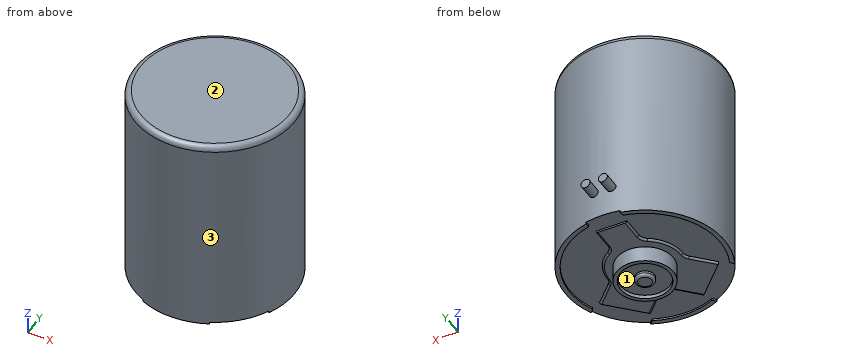
from build123d import *

# Parameters (mm, degrees)
SKETCH_1_R          = 21.05
EXTRUDE_1_DEPTH     = 53.3
FILLET_1_R          = 1.5
CUT_EXTRUDE_1_DEPTH = 0.5
SKETCH_3_R          = 7.5
EXTRUDE_2_DEPTH     = 4.2
SKETCH_4_R          = 6.5
CUT_EXTRUDE_2_DEPTH = 1
SKETCH_5_R          = 2.5
EXTRUDE_3_DEPTH     = 1.3
FILLET_2_R          = 0.75
FILLET_3_R          = 2.5
FILLET_4_R          = 0.5
SKETCH_7_W          = 9
SKETCH_7_H          = 4.55
CUT_EXTRUDE_3_DEPTH = 0.5
SKETCH_9_R          = 21
EXTRUDE_4_DEPTH     = 39.2
EXTRUDE_5_DEPTH     = 2
SKETCH_11_R         = 8
EXTRUDE_6_DEPTH     = 0.5
SKETCH_12_R         = 7.1
EXTRUDE_7_DEPTH     = 1
SKETCH_13_R         = 4
EXTRUDE_8_DEPTH     = 20
SKETCH_14_W         = 8
SKETCH_14_H         = 12
CUT_EXTRUDE_4_DEPTH = 1
SKETCH_15_R         = 2
CUT_EXTRUDE_5_DEPTH = 6
CHAMFER_1_SIZE      = 0.5
EXTRUDE_9_DEPTH     = 25
CHAMFER_2_SIZE      = 0.2
OTHER_START         = 53.3
OTHER_1_OUTLINE_R   = 21
OTHER_1_DEPTH       = 61.2


# Read off the part's stored shape, not the designer's step: 交差1
with BuildPart() as part:
    # ｽｹｯﾁ1 → ﾎﾞｽ - 押し出し1 (new body)
    with BuildSketch(Plane.XY):
        Circle(SKETCH_1_R)
    extrude(amount=EXTRUDE_1_DEPTH)

    # ﾌｨﾚｯﾄ1
    fillet_1_edges = [part.edges().sort_by_distance(p)[0] for p in [
        (-21.05, 0, 53.3),
    ]]
    fillet(fillet_1_edges, radius=FILLET_1_R)

    # ｽｹｯﾁ2 → ｶｯﾄ - 押し出し1 (cut)
    with BuildSketch(Plane(origin=(0, 0, 0), x_dir=(-1, 0, 0), z_dir=(0, 0, -1))):
        with BuildLine():
            Line((-1.767766953, -10.606601718), (-8.902744604, -17.741579369))
            ThreePointArc((-8.902744604, -17.741579369), (0, -19.85), (8.902744604, -17.741579369))
            Line((8.902744604, -17.741579369), (1.767766953, -10.606601718))
            ThreePointArc((1.767766953, -10.606601718), (0, -9.874368671), (-1.767766953, -10.606601718))
        make_face()
        with BuildLine():
            Line((-17.741579369, -8.902744604), (-9.939267924, -1.100433159))
            ThreePointArc((-9.939267924, -1.100433159), (-8.682968675, 4.960449072), (-4.1, 9.120855223))
            Line((-4.1, 9.120855223), (-4.1, 19.421959221))
            ThreePointArc((-4.1, 19.421959221), (-17.883955352, 8.613166721), (-17.741579369, -8.902744604))
        make_face()
        with BuildLine():
            Line((4.1, 19.421959221), (4.1, 9.120855223))
            ThreePointArc((4.1, 9.120855223), (8.682968675, 4.960449072), (9.939267924, -1.100433159))
            Line((9.939267924, -1.100433159), (17.741579369, -8.902744604))
            ThreePointArc((17.741579369, -8.902744604), (17.883955352, 8.613166721), (4.1, 19.421959221))
        make_face()
    extrude(amount=-CUT_EXTRUDE_1_DEPTH, mode=Mode.SUBTRACT)

    # ｽｹｯﾁ3 → ﾎﾞｽ - 押し出し2 (add)
    with BuildSketch(Plane(origin=(0, 0, 0), x_dir=(-1, 0, 0), z_dir=(0, 0, -1))):
        with Locations(Location((0, 0, 0), (0, 0, 180))):
            Circle(SKETCH_3_R)
    extrude(amount=EXTRUDE_2_DEPTH)

    # ｽｹｯﾁ4 → ｶｯﾄ - 押し出し2 (cut)
    with BuildSketch(Plane(origin=(0, 0, -4.2), x_dir=(-1, 0, 0), z_dir=(0, 0, -1))):
        Circle(SKETCH_4_R)
    extrude(amount=-CUT_EXTRUDE_2_DEPTH, mode=Mode.SUBTRACT)

    # ｽｹｯﾁ5 → ﾎﾞｽ - 押し出し3 (add)
    with BuildSketch(Plane(origin=(0, 0, -3.2), x_dir=(-1, 0, 0), z_dir=(0, 0, -1))):
        Circle(SKETCH_5_R)
    extrude(amount=EXTRUDE_3_DEPTH)

    # ﾌｨﾚｯﾄ2
    fillet_2_edges = [part.edges().sort_by_distance(p)[0] for p in [
        (2.5, 0, -4.5),
    ]]
    fillet(fillet_2_edges, radius=FILLET_2_R)

    # ﾌｨﾚｯﾄ3
    fillet_3_edges = [part.edges().sort_by_distance(p)[0] for p in [
        (-9.939267924, -1.100433159, 0.25),
        (-4.1, 9.120855223, 0.25),
        (4.1, 9.120855223, 0.25),
        (9.939267924, -1.100433159, 0.25),
    ]]
    fillet(fillet_3_edges, radius=FILLET_3_R)

    # ﾌｨﾚｯﾄ4
    fillet_4_edges = [part.edges().sort_by_distance(p)[0] for p in [
        (5.335255779, -14.174090543, 0),
        (-5.335255779, -14.174090543, 0),
        (-14.236593669, -5.397758904, 0),
        (-10.184921124, -1.070153656, 0),
        (-8.764891514, 4.814216109, 0),
        (-4.414822662, 9.401058845, 0),
        (14.236593669, -5.397758904, 0),
        (10.184921124, -1.070153656, 0),
        (8.764891514, 4.814216109, 0),
        (4.414822662, 9.401058845, 0),
        (0, -9.874368671, 0),
        (-4.1, 15.018756923, 0),
        (4.1, 15.018756923, 0),
    ]]
    fillet(fillet_4_edges, radius=FILLET_4_R - 0.0001)  # a hair under: the kernel refuses the full size

    # ｽｹｯﾁ7 → ｶｯﾄ - 押し出し3 (cut)
    with BuildSketch(Plane(origin=(0, 0, 0), x_dir=(-1, 0, 0), z_dir=(0, 0, -1))):
        with Locations((0, 18.775)):
            Rectangle(SKETCH_7_W, SKETCH_7_H)
        Polygon((-6.257895014, -16.510943341), (-9.75807358, -20.011121908), (-20.011121908, -9.75807358), (-16.510943341, -6.257895014), align=None)
        Polygon((6.257895014, -16.510943341), (16.510943341, -6.257895014), (20.011121908, -9.75807358), (9.75807358, -20.011121908), align=None)
    extrude(amount=-CUT_EXTRUDE_3_DEPTH, mode=Mode.SUBTRACT)

    # ｽｹｯﾁ9 → ﾎﾞｽ - 押し出し4 (add)
    with BuildSketch(Plane.XY.offset(53.3)):
        Circle(SKETCH_9_R)
    extrude(amount=EXTRUDE_4_DEPTH)

    # ｽｹｯﾁ10 → ﾎﾞｽ - 押し出し5 (add)
    with BuildSketch(Plane.XY.offset(92.5)):
        with BuildLine():
            Line((4.667626369, 11.595829599), (11.595829599, 4.667626369))
            ThreePointArc((11.595829599, 4.667626369), (8.838834765, -8.838834765), (-4.667626369, -11.595829599))
            Line((-4.667626369, -11.595829599), (-11.595829599, -4.667626369))
            ThreePointArc((-11.595829599, -4.667626369), (-8.838834765, 8.838834765), (4.667626369, 11.595829599))
        make_face()
    extrude(amount=EXTRUDE_5_DEPTH)

    # ｽｹｯﾁ11 → ﾎﾞｽ - 押し出し6 (add)
    with BuildSketch(Plane.XY.offset(94.5)):
        Circle(SKETCH_11_R)
    extrude(amount=EXTRUDE_6_DEPTH)

    # ｽｹｯﾁ12 → ﾎﾞｽ - 押し出し7 (add)
    with BuildSketch(Plane.XY.offset(95)):
        Circle(SKETCH_12_R)
    extrude(amount=EXTRUDE_7_DEPTH)

    # ｽｹｯﾁ13 → ﾎﾞｽ - 押し出し8 (add)
    with BuildSketch(Plane.XY.offset(94.5)):
        Circle(SKETCH_13_R)
    extrude(amount=EXTRUDE_8_DEPTH)

    # ｽｹｯﾁ14 → ｶｯﾄ - 押し出し4 (cut)
    with BuildSketch(Plane(origin=(0, 4, 0), x_dir=(1, 0, 0), z_dir=(0, 1, 0))):
        with Locations((0, -108.5)):
            Rectangle(SKETCH_14_W, SKETCH_14_H)
    extrude(amount=-CUT_EXTRUDE_4_DEPTH, mode=Mode.SUBTRACT)

    # ｽｹｯﾁ15 → ｶｯﾄ - 押し出し5 (cut)
    with BuildSketch(Plane.XY.offset(92.5)):
        with Locations((0, 17.5)):
            Circle(SKETCH_15_R)
        with Locations((17.5, 0)):
            Circle(SKETCH_15_R)
        with Locations((0, -17.5)):
            Circle(SKETCH_15_R)
        with Locations((-17.5, 0)):
            Circle(SKETCH_15_R)
    extrude(amount=-CUT_EXTRUDE_5_DEPTH, mode=Mode.SUBTRACT)

    # 面取り1
    chamfer_1_edges = [part.edges().sort_by_distance(p)[0] for p in [
        (-21, 0, 53.3),
        (-21, 0, 92.5),
    ]]
    chamfer(chamfer_1_edges, length=CHAMFER_1_SIZE)

    # ｽｹｯﾁ19 → ﾎﾞｽ - 押し出し9 (add)
    with BuildSketch(Plane(origin=(0, 0, 0), x_dir=(1, 0, 0), z_dir=(0, 1, 0))):
        with BuildLine():
            add(Edge.make_bspline(
                [(-2.3, -9.3), (-2.141895722, -9.3), (-1.984582336, -9.26831111), (-1.695786007, -9.148505891), (-1.561830045, -9.059042657), (-1.339916148, -8.83681524), (-1.250815241, -8.703488676), (-1.130324814, -8.411202826), (-1.099488051, -8.254725269), (-1.100524759, -7.937433107), (-1.132539642, -7.780879651), (-1.254416503, -7.490445543), (-1.344667636, -7.357097524), (-1.567516387, -7.136655943), (-1.702165246, -7.047850886), (-1.991590037, -6.92982589), (-2.149326122, -6.899295567), (-2.461692814, -6.900729728), (-2.617940839, -6.932319306), (-2.907178904, -7.053148359), (-3.038602416, -7.141124571), (-3.26167511, -7.365046532), (-3.349599592, -7.497417785), (-3.469481665, -7.788427754), (-3.500435327, -7.946423907), (-3.499555239, -8.260305399), (-3.467445926, -8.418673048), (-3.34669763, -8.707376797), (-3.256905259, -8.840768765), (-3.035347061, -9.061077904), (-2.902667973, -9.149452405), (-2.612947139, -9.269026571), (-2.458104278, -9.3), (-2.3, -9.3)],
                knots=[0, 0, 0, 0, 0.0625, 0.0625, 0.125, 0.125, 0.1875, 0.1875, 0.25, 0.25, 0.3125, 0.3125, 0.375, 0.375, 0.4375, 0.4375, 0.5, 0.5, 0.5625, 0.5625, 0.625, 0.625, 0.6875, 0.6875, 0.75, 0.75, 0.8125, 0.8125, 0.875, 0.875, 0.9375, 0.9375, 1, 1, 1, 1], degree=3))
        make_face()
        with BuildLine():
            add(Edge.make_bspline(
                [(2.3, -9.3), (2.458101824, -9.3), (2.615002003, -9.268333612), (2.902663727, -9.149297919), (3.036114818, -9.060490649), (3.257502016, -8.83999811), (3.346925979, -8.707290324), (3.468262095, -8.416258156), (3.499849023, -8.259893759), (3.500149899, -7.94238048), (3.468784785, -7.78588338), (3.348388342, -7.495343893), (3.259144479, -7.362166602), (3.038513671, -7.141379213), (2.905239906, -7.052187197), (2.617888296, -6.932449554), (2.460768356, -6.900612609), (2.148510682, -6.899405329), (1.991426227, -6.92973338), (1.700237772, -7.048797353), (1.567538038, -7.136292434), (1.342020343, -7.360062317), (1.253313742, -7.492276634), (1.131817712, -7.783408851), (1.100245068, -7.941102293), (1.09975782, -8.255174381), (1.131152757, -8.41364744), (1.250962434, -8.703405981), (1.340590257, -8.837664202), (1.562488668, -9.059527262), (1.695817167, -9.148670082), (1.986527204, -9.268965629), (2.141898176, -9.3), (2.3, -9.3)],
                knots=[0, 0, 0, 0, 0.0625, 0.0625, 0.125, 0.125, 0.1875, 0.1875, 0.25, 0.25, 0.3125, 0.3125, 0.375, 0.375, 0.4375, 0.4375, 0.5, 0.5, 0.5625, 0.5625, 0.625, 0.625, 0.6875, 0.6875, 0.75, 0.75, 0.8125, 0.8125, 0.875, 0.875, 0.9375, 0.9375, 1, 1, 1, 1], degree=3))
        make_face()
    extrude(amount=EXTRUDE_9_DEPTH)

    # 面取り2
    chamfer_2_edges = [part.edges().sort_by_distance(p)[0] for p in [
        (-1.645751311, -3.645751311, 114.5),
    ]]
    chamfer(chamfer_2_edges, length=CHAMFER_2_SIZE)

    # 交差1 outline → 交差1 (cut)
    with BuildSketch(Plane.XY.offset(OTHER_START)):
        Circle(OTHER_1_OUTLINE_R)
    extrude(amount=OTHER_1_DEPTH, mode=Mode.SUBTRACT)


solid = part.part
Input: part model. Units: mm. Frame: model coordinates. Face numbers are marked on the shaded views. Round coordinates to 2 decimals unless told otherwise and drop trailing zeros. Loops run counter-clockwise (first coordinate to the right, second up) from the corner with the lowest first, then second, coordinate; pieces in that order, holes last. Notation, with made-up numbers: (5, 87.5) -> (17, 87.5) arc R16 ccw to (17, 96.5) -> close; hole circle Ø3 at (18, 55). An arc over 180 degrees is marked (long way). Answer as a JSON object with one key per item and string values. Group by question number.
1) Section query B-B on z = 32.5. Output: boundary loops of the cut face in (x, y), plus the area to 3 significant figures.
2) Pin query (flat end, axial travel): pin 1 (13 mm diameter, centred on x = -10, y = 8.5, fed in from -Z); pin 2 (1 mm diameter, centred on x = 13, z = 23.5, fed in from +Y); pin 3 (1 mm diameter, centred on x = 1.5, z = 4.5, fed in from -Y). Return the tip coordinate at first contact, or that it passes through.
3) Ray query, L1, parallel to Y at x = 0, z = -3.65; L2, parallel to Z at x = 3, y = 15.5; L3, parallel to Z at x = -11, y = -14.5. Return the intervals inside material, ascending.
4) Draft query along Y for the marked faces 1, 2 and 3. Return one class per face: +Y half, -Y half, draft (parallel to the pull), parting line (faces both ways), or undercut.
Reply:
{
 "1": {"outline": "circle Ø42.1 at (0, 0)", "area": "1,390 mm2"},
 "2": {"pin 1": "stops at z = -4.2", "pin 2": "stops at y = 16.94", "pin 3": "stops at y = -21.03"},
 "3": {"L1": "y = -7.5 to -6.5, -2.5 to 2.5, 6.5 to 7.5", "L2": "z = 0 to 53.3", "L3": "z = 0.5 to 53.3"},
 "4": {"face 1": "undercut", "face 2": "draft", "face 3": "parting line"}
}
